```python
from build123d import *

# Parameters (mm, degrees)
SKETCH1_W           = 35
SKETCH1_H           = 28
SKETCH1_R           = 2
BOSS_EXTRUDE1_DEPTH = 28.5
SKETCH2_R           = 4
CUT_EXTRUDE1_DEPTH  = 54.115440316


with BuildPart() as part:
    # Sketch1 → Boss-Extrude1 (new body)
    with BuildSketch(Plane.XY):
        with Locations((17.5, 14)):
            Rectangle(SKETCH1_W, SKETCH1_H)
        with Locations(Location((5.5, 22.5, 0), (0, 0, 180))):
            Circle(SKETCH1_R, mode=Mode.SUBTRACT)
        with Locations(Location((29.5, 22.5, 0), (0, 0, 180))):
            Circle(SKETCH1_R, mode=Mode.SUBTRACT)
        with Locations(Location((5.5, 5.5, 0), (0, 0, 180))):
            Circle(SKETCH1_R, mode=Mode.SUBTRACT)
        with Locations(Location((29.5, 5.5, 0), (0, 0, 180))):
            Circle(SKETCH1_R, mode=Mode.SUBTRACT)
    extrude(amount=BOSS_EXTRUDE1_DEPTH)

    # Sketch2 → Cut-Extrude1 (cut, through all)
    with BuildSketch(Plane.XZ):
        with Locations((17.5, 14.25)):
            Circle(SKETCH2_R)
    extrude(amount=-CUT_EXTRUDE1_DEPTH, mode=Mode.SUBTRACT)


solid = part.part
```
Verification items for the finished model (mm, model axes). Round coordinates to 2 decimals unless told otherwise and drop trailing zeros. Loops run counter-clockwise (first coordinate to the right, second up) from the corner with the lowest first, then second, coordinate; pieces in that order, holes last. Notation, with made-up numbers: (-21.5, 70) -> (-9.5, 70) arc R7 cw to (-9.5, 80) -> close; hole circle Ø10 at (13, 38). An arc over 180 degrees is marked (long way). Answer as a JSON object with one key per item and string values.
Q1. Section check B-B (x = 17.5). Record the boundary of the cut face in (y, z), then the cut area to 3 significant figures.
Data:
{"outline": "(0, 0) -> (28, 0) -> (28, 10.25) -> (0, 10.25) -> close; (0, 18.25) -> (28, 18.25) -> (28, 28.5) -> (0, 28.5) -> close", "area": "574 mm2"}
Q2. Section check D-D (x = 5.5). Record the boundary of the cut face in (y, z).
Data:
{"outline": "(0, 0) -> (3.5, 0) -> (3.5, 28.5) -> (0, 28.5) -> close; (7.5, 0) -> (20.5, 0) -> (20.5, 28.5) -> (7.5, 28.5) -> close; (24.5, 0) -> (28, 0) -> (28, 28.5) -> (24.5, 28.5) -> close"}
Q3. Section check C-C (y = 17.25). Record the boundary of the cut face in (x, z), then the cut area to 3 significant figures.
Data:
{"outline": "(0, 0) -> (35, 0) -> (35, 28.5) -> (0, 28.5) -> close; hole circle Ø8 at (17.5, 14.25)", "area": "947 mm2"}
Q4. Section check A-A (z = 14.25). Record the boundary of the cut face in (x, y).
Data:
{"outline": "(0, 0) -> (13.5, 0) -> (13.5, 28) -> (0, 28) -> close; (21.5, 0) -> (35, 0) -> (35, 28) -> (21.5, 28) -> close; hole circle Ø4 at (5.5, 5.5); hole circle Ø4 at (5.5, 22.5); hole circle Ø4 at (29.5, 5.5); hole circle Ø4 at (29.5, 22.5)"}
Q5. Go/stop test with a flat-tipped pin: P1, Ø10, axis at y = 3, z = 20, coming from the -X side. Record where the tip stops, or that it passes through.
Data:
{"P1": "stops at x = 0"}
Q6. Scan lines: line 1 (Y direction, x = 5.5, z = 19); line 2 (Y direction, x = 7, z = 10); line 3 (X direction, y = 23.75, z = 22.75). Record each from-to range of solid material in increasing order. Write a range as from..to.
Data:
{"line 1": "y = 0..3.5, 7.5..20.5, 24.5..28", "line 2": "y = 0..4.18, 6.82..21.18, 23.82..28", "line 3": "x = 0..3.94, 7.06..27.94, 31.06..35"}
Q7. Draft check along X on faces 1 (the flat face through (0, 14, 14)), 2 (the cylindrical face through (14.55, 13.8, 16.95)), 3 (the flat face through (13, 0, 14)). Enter one of: pulls with the +X half, pulls with the -X half, needs draft (parallel to the pull), parting line crosses it, or undercut.
Data:
{"face 1": "pulls with the -X half", "face 2": "undercut", "face 3": "needs draft"}
